Part model, mm, in its own coordinate system. Face numbers are marked on the shaded views. Coordinates: 2 decimals unless noted, no trailing zeros. Write each loop counter-clockwise with the first axis right and the second up, starting at its lowest first coordinate (ties: lowest second). Pieces come first, ordered by that corner, then holes. Notation, with made-up numbers: (44.25, 80.5) - (80.25, 80.5) arc R17 ccw to (80.25, 88.5) - close; hole circle Ø1 at (67.25, 86.25). An arc over 180 degrees is marked (long way). Use one line per item in the form item = value. Start each with the question number.
from build123d import *

# Parameters (mm, degrees)
EXTRUDE_1_DEPTH     = 100
CUT_EXTRUDE_1_DEPTH = 102.662431606
SKETCH_3_W          = 21
SKETCH_3_H          = 2
EXTRUDE_2_DEPTH     = 10
SKETCH_4_R          = 1.5
EXTRUDE_3_DEPTH     = 2


with BuildPart() as part:
    # Эскиз1 → Бобышка-Вытянуть1 (new body)
    with BuildSketch(Plane.XY):
        Polygon((0, 0), (-8.5, 0), (-8.5, 15), (-10.5, 15), (-10.5, -2), (10.5, -2), (10.5, 15), (8.5, 15), (8.5, 0), align=None)
    extrude(amount=EXTRUDE_1_DEPTH)

    # Эскиз2 → Вырез-Вытянуть1 (cut, through all)
    with BuildSketch(Plane(origin=(0, 0, 0), x_dir=(1, 0, 0), z_dir=(0, 1, 0))):
        Polygon((0, -15), (-8.5, -15), (-8.5, -40), (8.5, -40), (8.5, -15), align=None)
    extrude(amount=-CUT_EXTRUDE_1_DEPTH, mode=Mode.SUBTRACT)

    # Эскиз3 → Бобышка-Вытянуть2 (add)
    with BuildSketch(Plane(origin=(0, 0, 0), x_dir=(-1, 0, 0), z_dir=(0, 0, -1))):
        with Locations((0, 16)):
            Rectangle(SKETCH_3_W, SKETCH_3_H)
    extrude(amount=-EXTRUDE_2_DEPTH)

    # Эскиз4 → Бобышка-Вытянуть3 (add)
    # profile 1 of 2: a face of its own
    with BuildSketch(Plane(origin=(0, 0, 0), x_dir=(-1, 0, 0), z_dir=(0, 0, -1))):
        Polygon((-3.5, 27.5), (3.5, 27.5), (3.5, 20.5), (3.5, 17), (0, 17), (-3.5, 17), (-3.5, 20.5), align=None)
        with Locations((0, 24)):
            Circle(SKETCH_4_R, mode=Mode.SUBTRACT)
    # profile 2 of 2: a face of its own
    with BuildSketch(Plane(origin=(0, 0, 0), x_dir=(-1, 0, 0), z_dir=(0, 0, -1))):
        Polygon((3.5, -3.5), (3.5, -10.5), (-3.5, -10.5), (-3.5, -3.5), (-3.5, -2), (0, -2), (3.5, -2), align=None)
        with Locations((0, -7)):
            Circle(SKETCH_4_R, mode=Mode.SUBTRACT)
    extrude(amount=-EXTRUDE_3_DEPTH)


solid = part.part
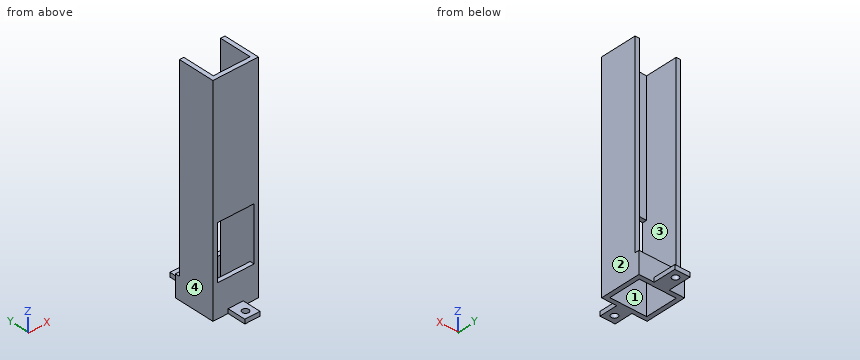
Q1. Mould opens along X. For the marked faces 1, 2, 3 and 4 say: released by +X, released by -X, zero draft, split by the parting line, or undercut.
Q2. Slice it at B-B (x = 0). List the corners of the cut face in (y, z), plus the area to 3 significant figures.
Q3. Slice it at A-A (y = 12). List the corners of the cut face in (x, z), plus the area to 3 significant figures.
Q4. Pin check, flat tips, straight feed: P1, Ø8.5, axis at x = -2, z = 82, coming from the +Y side; P2, Ø1, axis at y = -8, z = 1.5, coming from the +X side; P3, Ø10, axis at x = 7.5, z = 22.5, coming from the +Y side; P4, Ø6.5, axis at x = -3, z = 35, coming from the -Y side. Stop position of each tip, or through.
Q5. Drill centre lines: probe 1 along Y at (x, z) = (0, 1.65); probe 2 along X at (y, z) = (11, 94.5); probe 3 along Z at (x, y) = (4.5, -1). Where is each one in solid material? Low to high.
Q6. Slice it at D-D (x = 6.5). List the corners of the cut face in (y, z), plus the area to 3 significant figures.
Q7. Slice it at C-C (z = 20). List the corners of the cut face in (x, y).
Solution:
q1.face_1 = undercut
q1.face_2 = released by +X
q1.face_3 = undercut
q1.face_4 = released by -X
q2.outline = (-10.5, 0) - (-8.5, 0) - (-8.5, 2) - (-10.5, 2) - close; (-5.5, 0) - (0, 0) - (0, 15) - (-2, 15) - (-2, 2) - (-5.5, 2) - close; (-2, 40) - (0, 40) - (0, 100) - (-2, 100) - close; (15, 0) - (22.5, 0) - (22.5, 2) - (17, 2) - (17, 10) - (15, 10) - close; (25.5, 0) - (27.5, 0) - (27.5, 2) - (25.5, 2) - close
q2.area = 196 mm2
q3.outline = (-10.5, 0) - (-8.5, 0) - (-8.5, 100) - (-10.5, 100) - close; (8.5, 0) - (10.5, 0) - (10.5, 100) - (8.5, 100) - close
q3.area = 400 mm2
q4.P1 = 0
q4.P2 = 3.5
q4.P3 = 15
q4.P4 = through
q5.probe_1 = -10.5 to -8.5, -5.5 to 0, 15 to 22.5, 25.5 to 27.5
q5.probe_2 = -10.5 to -8.5, 8.5 to 10.5
q5.probe_3 = 0 to 15, 40 to 100
q6.outline = (-2, 0) - (0, 0) - (0, 15) - (-2, 15) - close; (-2, 40) - (0, 40) - (0, 100) - (-2, 100) - close; (15, 0) - (17, 0) - (17, 10) - (15, 10) - close
q6.area = 170 mm2
q7.outline = (-10.5, -2) - (-8.5, -2) - (-8.5, 15) - (-10.5, 15) - close; (8.5, -2) - (10.5, -2) - (10.5, 15) - (8.5, 15) - close
